Solid Edge part; units mm, degrees
sketch "Sketch1" plane through (0, 0, 0) normal (0, 0, 1) x (1, 0, 0)
  line L0 (22.7, 13.5) -> (-22.7, 13.5)
  line L1 (-22.7, 13.5) -> (-22.7, -13.5)
  line L2 (-22.7, -13.5) -> (22.7, -13.5)
  line L3 (22.7, -13.5) -> (22.7, 13.5)
extrude "Protrusion1" add sketch "Sketch1" along normal blind 5
sketch "Sketch2" plane through (0, 0, 0) normal (1, 0, 0) x (0, 1, 0)
  line L0 (13.5, 7) -> (17.5, 7)
  line L1 (17.5, 7) -> (17.5, -13)
  line L2 (17.5, -13) -> (13.5, -13)
  line L3 (13.5, -13) -> (13.5, 7)
  dimension "D1" = 17.5
extrude "Protrusion2" add sketch "Sketch2" along normal mid plane 45.4
hole "Hole_1" at (-10, 10, 5) direction (0, 0, -1) diameter 3.2 end up to next countersink diameter 6.94 countersink angle 90
pattern_linear "Pattern1" count 2 spacing 20 along (1, 0, 0) count 2 spacing 20 along (0, -1, 0) of "Hole_1"
Design review of the part built by this model. Coordinates are the model's own, in mm. A direction names the side the tool comes from. Round coordinates to 2 decimals unless told otherwise and drop trailing zeros. Write each loop counter-clockwise with the first axis right and the second up, starting at its lowest first coordinate (ties: lowest second). Pieces come first, ordered by that corner, then holes. Notation, with made-up numbers: M 75,68 L 134,68 A21 ccw 134,96 Z; hole C -26,16.5 d9. An arc over 180 degrees is marked long. One line per item, written item: value. Start each with the question number.
1. Take a section at B-B on x = 10. State how many separate pieces and enclosed holes the cut face has, then the cut area to 3 significant figures.
2. Take a section at A-A on y = -10. State the section outline as (x, z) points, then the cut area to 3 significant figures.
3. Take a section at C-C on z = 3.75. State the section outline as (x, y) points, then the cut area to 3 significant figures.
4. For faces 5 (the face through (22.7, 7, 1)), 6 (the face through (0, 13.5, -7)), 7 (the face through (0, 0, 5)), list the 3-axis set-ups (+Z, -Z, +X, -X, +Y, -Y) from which the entire face can be reached by the end or side of a thin tool; tool diameter is ignored.
5. Take a section at D-D on x = 4. State the section outline as (y, z) points, then the cut area to 3 significant figures.
6. Clearance check with flat-ended pins moving along their axes: P1, Ø10, axis at x = 2.5, y = 1, coming from the +Z side; P2, Ø3.5, axis at x = -10, y = 10, coming from the +Z side; P3, Ø1.5, axis at x = 10.5, y = 4.5, coming from the -Z side. State where each tip first meets the part, or that it passes through.
7. Draft analysis for pull direction Y (two halves, no side actions). For faces 1 (the face through (0, 16, -13)), 2 (the face through (10.07, -8.4, 1.59)), 3 (the face through (0, -13.5, 2)), 4 (the face through (-11.68, -9.63, 3.25)), state which applies: pulls with the +Y half, pulls with the -Y half, needs draft (parallel to the pull), parting line crosses it, or undercut.
8. To check wall thickness, follow probe 1 along Y at (x, z) = (10, 2.4); probe 2 along X at (y, z) = (10, 2.1); probe 3 along Y at (x, z) = (-3, -9.25). State the ranges of each line that lie inside material, in increasing order. Write a range as from..to.
Computed:
1. separate pieces: 3
1. enclosed holes: 0
1. area: 176 mm²
2. outline: M -22.7,0 L -11.6,0 L -11.6,3.13 L -13.47,5 L -22.7,5 Z; M -8.4,0 L 8.4,0 L 8.4,3.13 L 6.53,5 L -6.53,5 L -8.4,3.13 Z; M 11.6,0 L 22.7,0 L 22.7,5 L 13.47,5 L 11.6,3.13 Z
2. area: 188 mm²
3. outline: M -22.7,-13.5 L 22.7,-13.5 L 22.7,17.5 L -22.7,17.5 Z; hole C -10,-10 d4.44; hole C -10,10 d4.44; hole C 10,-10 d4.44; hole C 10,10 d4.44
3. area: 1,350 mm²
4. face 5: +Z, -Z, +X, +Y, -Y
4. face 6: -Z, +X, -X, -Y
4. face 7: +Z, +X, -X, -Y
5. outline: M -13.5,0 L 13.5,0 L 13.5,-13 L 17.5,-13 L 17.5,7 L 13.5,7 L 13.5,5 L -13.5,5 Z
5. area: 215 mm²
6. P1: stops at z = 5
6. P2: stops at z = 3.28
6. P3: stops at z = 0
7. face 1: needs draft
7. face 2: undercut
7. face 3: pulls with the -Y half
7. face 4: undercut
8. probe 1: y = -13.5..-11.6, -8.4..8.4, 11.6..17.5
8. probe 2: x = -22.7..-11.6, -8.4..8.4, 11.6..22.7
8. probe 3: y = 13.5..17.5
